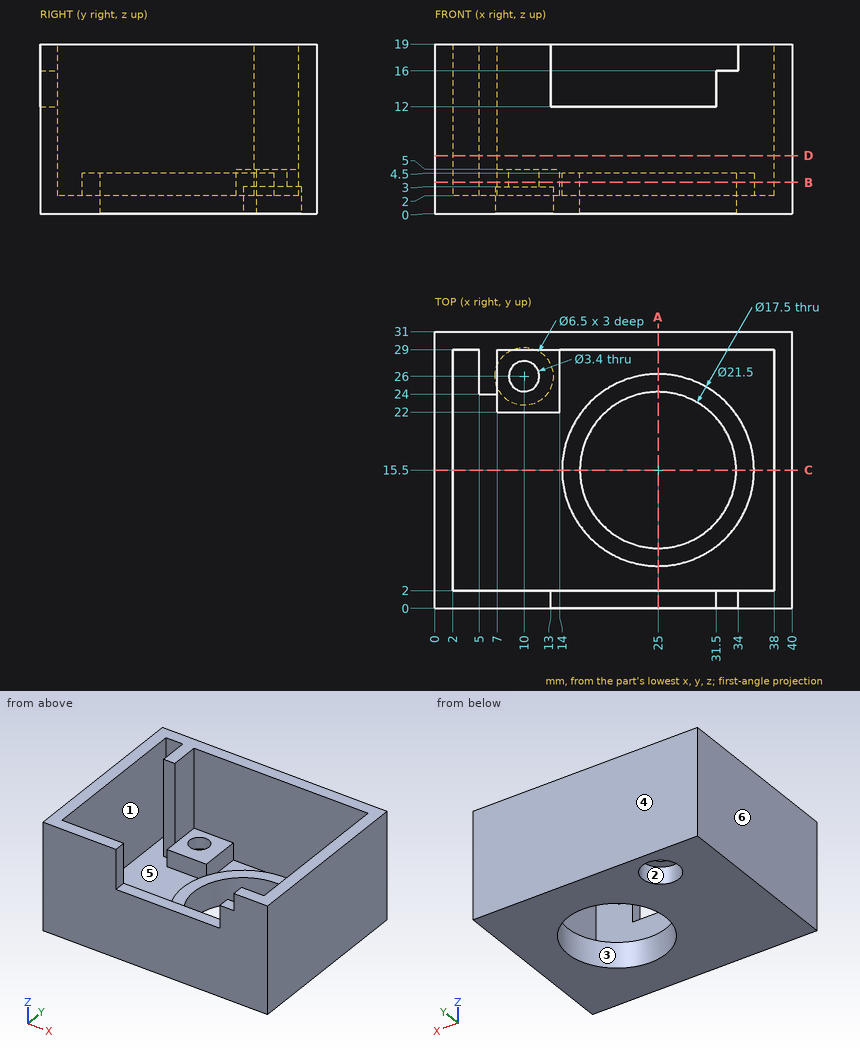
Could you check a few things on this drawing? It's one solid part, dimensions in mm from its lowest x, y, z. A direction names the side the tool comes from. Coordinates: 2 decimals unless noted, no trailing zeros. Order: outer loops, then holes, each group sorted by start corner. A loop starts at its lowest first (then second) coordinate and runs counter-clockwise, first axis right, second up.
1. For the marked faces 1, 2 and 3, which set-ups out of +Z, -Z, +X, -X, +Y, -Y let a thin tool reach every point of the face, with its end or its side?
2. If we section it at A-A (x = 25): Please give me the cut outline in (y, z), then the cut area to 3 significant figures.
3. If we section it at B-B (z = 3.5): Please give me the cut outline in (x, y), then the cut area to 3 significant figures.
4. I'm going to push flat-ended pins straight in: pin 1 (0.6 mm diameter, centred on x = 19, y = 1, fed in from +Z); pin 2 (1 mm diameter, centred on x = 29.5, y = 9, fed in from -Z); pin 3 (2 mm diameter, centred on x = 9, y = 26, fed in from +Z); pin 4 (1 mm diameter, centred on x = 32.5, y = 1, fed in from +Z). Where does each tip first touch, or does it pass through?
5. If we section it at D-D (z = 6.5): Please give me the cut outline in (x, y), then the cut area to 3 significant figures.
6. If we section it at C-C (y = 15.5): Please give me the cut outline in (x, z), then the cut area to 3 significant figures.
7. I need wall thicknesses on line 1 (Y direction, x = 25, z = 2.6); line 2 (X direction, y = 26.5, z = 13); line 3 (X direction, y = 23, z = 6.5). Which ranges of each line are inside material? Lowest first, please.
8. Thinking about a two-plate mould opening in X: for the marked faces 4, 5 and 6, which applies, +X half, -X half, draft (parallel to the pull), parting line (faces both ways), or undercut?
Entries:
1. face 1: +Z
1. face 2: -Z
1. face 3: +Z, -Z
2. outline: (0, 0) - (6.75, 0) - (6.75, 4.5) - (4.75, 4.5) - (4.75, 2) - (2, 2) - (2, 12) - (0, 12) - close; (24.25, 0) - (31, 0) - (31, 19) - (29, 19) - (29, 2) - (26.25, 2) - (26.25, 4.5) - (24.25, 4.5) - close
2. area: 91.0 mm2
3. outline: (0, 0) - (40, 0) - (40, 31) - (0, 31) - close; circle Ø21.5 at (25, 15.5); hole (2, 2) - (38, 2) - (38, 29) - (14, 29) - (14, 22) - (7, 22) - (7, 24) - (5, 24) - (5, 29) - (2, 29) - close; hole circle Ø3.4 at (10, 26); hole circle Ø17.5 at (25, 15.5)
3. area: 440 mm2
4. pin 1: stops at z = 12
4. pin 2: passes through
4. pin 3: stops at z = 5
4. pin 4: stops at z = 16
5. outline: (0, 0) - (40, 0) - (40, 31) - (0, 31) - close; hole (2, 2) - (38, 2) - (38, 29) - (7, 29) - (7, 24) - (5, 24) - (5, 29) - (2, 29) - close
5. area: 278 mm2
6. outline: (0, 0) - (16.25, 0) - (16.25, 4.5) - (14.25, 4.5) - (14.25, 2) - (2, 2) - (2, 19) - (0, 19) - close; (33.75, 0) - (40, 0) - (40, 19) - (38, 19) - (38, 2) - (35.75, 2) - (35.75, 4.5) - (33.75, 4.5) - close
6. area: 123 mm2
7. line 1: y = 0 to 2, 4.75 to 6.75, 24.25 to 26.25, 29 to 31
7. line 2: x = 0 to 2, 5 to 7, 38 to 40
7. line 3: x = 0 to 2, 38 to 40
8. face 4: draft
8. face 5: undercut
8. face 6: -X half
